Part model, mm, in its own coordinate system. Give positions to 0.01 mm unless a question says otherwise; leave off trailing zeros. Order: outer loops, then holes, each group sorted by start corner. A loop starts at its lowest first (then second) coordinate and runs counter-clockwise, first axis right, second up. Notation, with made-up numbers: M 67,-2 L 102,-2 A23 ccw 102,25 Z; hole C 18.5,-21 d9. An arc over 180 degrees is marked long. Write each question's results on one line, items separated by ' | '. Start each with the question number.
from build123d import *

# Parameters (mm, degrees)
SKETCH1_W           = 581.59
SKETCH1_H           = 272
BOSS_EXTRUDE1_DEPTH = 2
SKETCH2_W           = 400
SKETCH2_H           = 2.5
CUT_EXTRUDE1_DEPTH  = 10
CAVITY2_OUTLINE_W   = 10
CAVITY2_OUTLINE_H   = 2
CAVITY2_DEPTH       = 449.999196591


# Read off the part's stored shape, not the designer's step: Cavity2
with BuildPart() as part:
    # Sketch1 → Boss-Extrude1 (new body)
    with BuildSketch(Plane.XY):
        with Locations((290.795, 136)):
            Rectangle(SKETCH1_W, SKETCH1_H)
    extrude(amount=BOSS_EXTRUDE1_DEPTH)

    # Sketch2 → Cut-Extrude1 (cut)
    with BuildSketch(Plane(origin=(0, 0, 0), x_dir=(-1, 0, 0), z_dir=(0, 0, -1))):
        with Locations((-381.59, 17.25)):
            Rectangle(SKETCH2_W, SKETCH2_H)
    extrude(amount=-CUT_EXTRUDE1_DEPTH, mode=Mode.SUBTRACT)

    # Cavity2 outline → Cavity2 (cut)
    with BuildSketch(Plane.YZ):
        with Locations((5, 1)):
            Rectangle(CAVITY2_OUTLINE_W, CAVITY2_OUTLINE_H)
    extrude(amount=CAVITY2_DEPTH, mode=Mode.SUBTRACT)


solid = part.part
(1) Saw through at C-C on x = 101. Give the cut face in (y, z).
(2) Probe L1, parallel to Y at x = 372.5, z = 0.85; L2, parallel to Y at x = 453, z = 1.8; L3, parallel to Y at x = 48.5, z = 0.2. List the from-to ranges inside material, lowest first.
(3) Saw through at A-A on x = 409. Give the cut face in (y, z), plus the area to 3 significant figures.
(4) Drop flat-ended pins along their axis: P1, Ø1, axis at x = 234, z = 1, coming from the -Y side; P2, Ø0.6, axis at y = 17, z = 1.5, coming from the +X side. Give the stop position or say it passes through.
(5) Saw through at B-B on z = 0.6. Give the cut face in (x, y).
Taken from the geometry:
1) outline: M 10,0 L 272,0 L 272,2 L 10,2 Z
2) L1: y = 10 to 16, 18.5 to 272 | L2: y = 0 to 16, 18.5 to 272 | L3: y = 10 to 272
3) outline: M 10,0 L 16,0 L 16,2 L 10,2 Z; M 18.5,0 L 272,0 L 272,2 L 18.5,2 Z | area: 519 mm²
4) P1: stops at y = 10 | P2: stops at x = 181.59
5) outline: M 0,10 L 450,10 L 450,0 L 581.59,0 L 581.59,16 L 181.59,16 L 181.59,18.5 L 581.59,18.5 L 581.59,272 L 0,272 Z
